from build123d import *

# Parameters (mm, degrees)
EXTRUDE_1_DEPTH = 10
EXTRUDE_5_DEPTH = 10
EXTRUDE_START   = 10
SKETCH_5_R      = 5
EXTRUDE_6_DEPTH = 10


with BuildPart() as part:
    # 草图1 → 凸台-拉伸1 (new body)
    with BuildSketch(Plane(origin=(0, 0, 0), x_dir=(1, 0, 0), z_dir=(0, 1, 0))):
        with BuildLine():
            ThreePointArc((-49.180194883, -49.180194883), (69.551298604, 0), (-49.180194883, 49.180194883))
            ThreePointArc((-49.180194883, 49.180194883), (-31.357669024, 0), (-49.180194883, -49.180194883))
        make_face()
        with BuildLine():
            Line((-2, 9.797958971), (-2, 13.797958971))
            Line((-2, 13.797958971), (2, 13.797958971))
            Line((2, 13.797958971), (2, 9.797958971))
            ThreePointArc((2, 9.797958971), (0, -10), (-2, 9.797958971))
        make_face(mode=Mode.SUBTRACT)
    extrude(amount=EXTRUDE_1_DEPTH)

    # 草图4 → 凸台-拉伸5 (add)
    with BuildSketch(Plane(origin=(0, 10, 0), x_dir=(1, 0, 0), z_dir=(0, 1, 0))):
        with BuildLine():
            Line((-80, 5), (-23.481338819, 5))
            Line((-23.481338819, 5), (-23.481338819, -5))
            Line((-23.481338819, -5), (-80, -5))
            ThreePointArc((-80, -5), (-85, 0), (-80, 5))
        make_face()
    extrude(amount=EXTRUDE_5_DEPTH)

    # 草图5 → 凸台-拉伸6 (add)
    with BuildSketch(Plane.XZ.offset(-10).offset(EXTRUDE_START)):
        with Locations(Location((-80, 0, 0), (0, 0, 270))):
            Circle(SKETCH_5_R)
    extrude(amount=-EXTRUDE_6_DEPTH)


solid = part.part
Geometry: final body of the model. Coordinates: model frame, mm. A direction names the side the tool comes from. Give positions to 0.01 mm unless a question says otherwise; leave off trailing zeros. Order: outer loops, then holes, each group sorted by start corner. A loop starts at its lowest first (then second) coordinate and runs counter-clockwise, first axis right, second up. Notation, with made-up numbers: (43, 55.25) -> (82, 55.25) arc R17 ccw to (82, 88.25) -> close; hole circle Ø9 at (0.25, 69.5). An arc over 180 degrees is marked (long way). Answer as a JSON object with one key per item and string values.
Q1. Section C-C (z = 0). Output: boundary loops of the cut face in (x, y), plus the area to 3 significant figures.
Entries:
{"outline": "(-85, 0) -> (-75, 0) -> (-75, 10) -> (-31.36, 10) -> (-31.36, 0) -> (-10, 0) -> (-10, 10) -> (-23.48, 10) -> (-23.48, 20) -> (-85, 20) -> close; (10, 0) -> (69.55, 0) -> (69.55, 10) -> (10, 10) -> close", "area": "1,520 mm^2"}
Q2. Material intervals for probe 1 along X at (y, z) = (6, 0); probe 2 along Z at (x, y) = (0, 4.25); probe 3 along Y at (x, z) = (-31, -24), sorted ascending.
Entries:
{"probe 1": "x = -85 to -75, -31.36 to -10, 10 to 69.55", "probe 2": "z = -69.55 to -13.8, 10 to 69.55", "probe 3": "y = 0 to 10"}
Q3. First-contact query: pin 1 (4.5 mm diameter, centred on x = 0, y = 6, fed in from +Z); pin 2 (1.5 mm diameter, centred on x = 25, z = 7.5, fed in from +Y); pin 3 (2 mm diameter, centred on y = 3.5, z = -33, fed in from -X). Flat tips, straight axial feed; report the tip coordinate or a pass-through.
Entries:
{"pin 1": "stops at z = 69.55", "pin 2": "stops at y = 10", "pin 3": "stops at x = -39.3"}
Q4. Section B-B (x = 0). Output: boundary loops of the cut face in (y, z).
Entries:
{"outline": "(0, -69.55) -> (10, -69.55) -> (10, -13.8) -> (0, -13.8) -> close; (0, 10) -> (10, 10) -> (10, 69.55) -> (0, 69.55) -> close"}
Q5. Access query for faces 1 (the flat face through (-2, 5, -12)), 2 (the flat face through (-54, 20, 0)), 3 (the flat face through (-55, 10, 0)), 4 (the flat face through (-23.481, 15, 0)), 5 (the flat face through (-80, 0, 0)). Directions: +Z, -Z, +X, -X, +Y, -Y. A direction counts if a zero-diameter tool reaches every point of the face in a straight line with its end or side. Return the directions, or none.
Entries:
{"face 1": "+Y, -Y", "face 2": "+Z, -Z, +X, -X, +Y", "face 3": "-Y", "face 4": "+Z, -Z, +X, +Y", "face 5": "+Z, -Z, +X, -X, -Y"}
Q6. Section D-D (x = -27.5). Output: boundary loops of the cut face in (y, z).
Entries:
{"outline": "(0, -63.88) -> (10, -63.88) -> (10, -5) -> (20, -5) -> (20, 5) -> (10, 5) -> (10, 63.88) -> (0, 63.88) -> close"}
Q7. Draft query along X for faces 6 (the flat face through (23, 0, -1)), 7 (the cylindrical face through (0, 5, 10)), 8 (the cylindrical face through (69.513, 4.93, 2.294)). Return one class per face: released by +X, released by -X, zero draft, split by the parting line, or undercut.
Entries:
{"face 6": "zero draft", "face 7": "undercut", "face 8": "split by the parting line"}
Q8. Section A-A (y = 6.5). Output: boundary loops of the cut face in (x, z).
Entries:
{"outline": "circle Ø10 at (-80, 0); (-49.18, -49.18) arc R69.55 ccw (long way) to (-49.18, 49.18) arc R76.77 cw to start; hole (-2, -13.8) -> (2, -13.8) -> (2, -9.8) arc R10 ccw (long way) to (-2, -9.8) -> close"}
